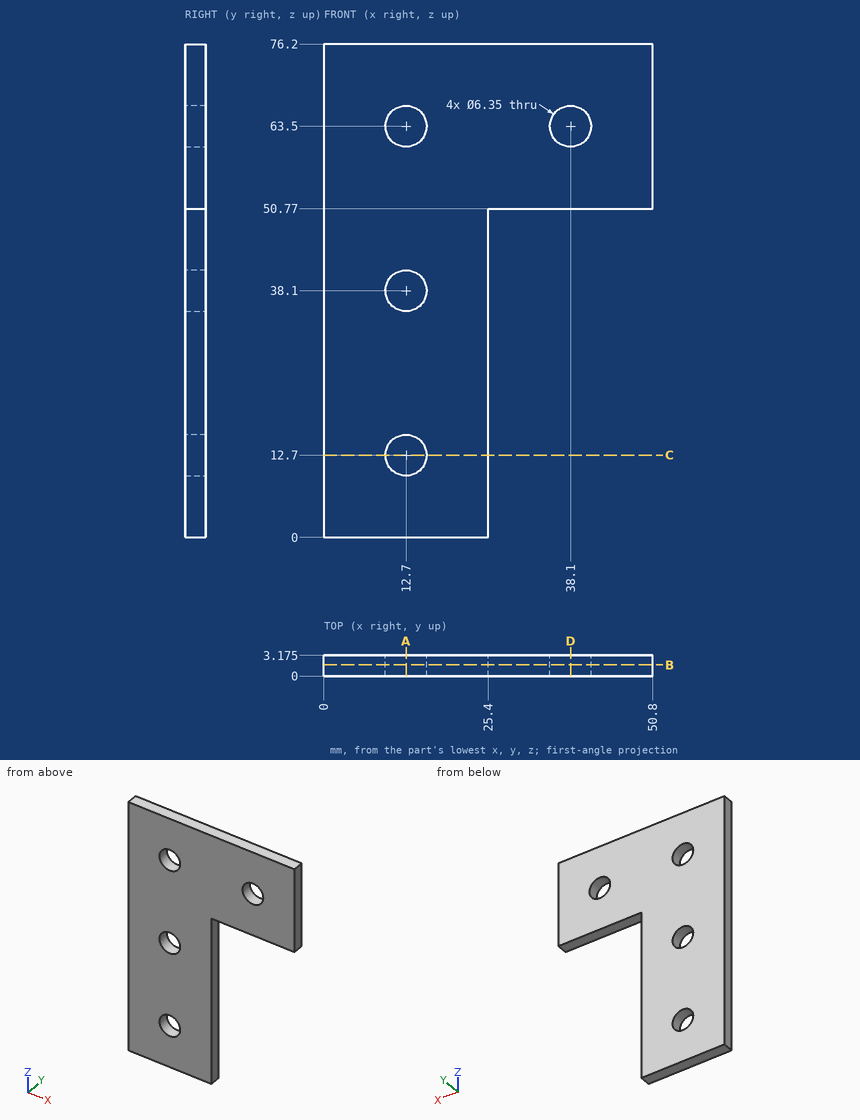
The drawing under review shows one solid part. Ordinate dimensions are in mm from its lowest x, y, z. Round coordinates to 2 decimals unless told otherwise and drop trailing zeros. Loops run counter-clockwise (first coordinate to the right, second up) from the corner with the lowest first, then second, coordinate; pieces in that order, holes last. Notation, with made-up numbers: (43.5, -29) - (92.5, -29) arc R34 cw to (92.5, 7) - close; hole circle Ø3 at (-35.5, 35.5). An arc over 180 degrees is marked (long way). One line per question, with ' | ' between items.
Q1. Take a section at B-B (y = 1.7). State how many separate pieces and enclosed holes the cut face has, and give its area (3 significant figures).
Taken from the geometry:
separate pieces: 1 | enclosed holes: 4 | area: 2,450 mm²
Q2. Take a section at C-C (z = 12.7). Give the boundary of the cut face in (x, y) (1 decimal).
Taken from the geometry:
outline: (0, 0) - (9.5, 0) - (9.5, 3.2) - (0, 3.2) - close; (15.9, 0) - (25.4, 0) - (25.4, 3.2) - (15.9, 3.2) - close
Q3. Take a section at D-D (x = 38.1). Give the boundary of the cut face in (y, z) (1 decimal).
Taken from the geometry:
outline: (0, 50.8) - (3.2, 50.8) - (3.2, 60.3) - (0, 60.3) - close; (0, 66.7) - (3.2, 66.7) - (3.2, 76.2) - (0, 76.2) - close
Q4. For line 1 along X through (y, z) = (0.85, 63.5) (1 decimal); line 2 along X through (y, z) = (1.7, 38.1) (1 decimal); line 3 along Z through (x, y) = (38.1, 2.4) (1 decimal), list the stretches that pass through material, from the lowest coordinate up. Write a range as [from, to].
Taken from the geometry:
line 1: x = [0, 9.5], [15.9, 34.9], [41.3, 50.8] | line 2: x = [0, 9.5], [15.9, 25.4] | line 3: z = [50.8, 60.3], [66.7, 76.2]
Q5. Take a section at A-A (x = 12.7). Give the boundary of the cut face in (y, z) (1 decimal).
Taken from the geometry:
outline: (0, 0) - (3.2, 0) - (3.2, 9.5) - (0, 9.5) - close; (0, 15.9) - (3.2, 15.9) - (3.2, 34.9) - (0, 34.9) - close; (0, 41.3) - (3.2, 41.3) - (3.2, 60.3) - (0, 60.3) - close; (0, 66.7) - (3.2, 66.7) - (3.2, 76.2) - (0, 76.2) - close
Q6. For pin 1 (1.5 mm diameter, centred on x = 33, z = 64.5, fed in from -Y); pin 2 (1.6 mm diameter, centred on y = 1, z = 19.5, fed in from +X), all flat-tipped, find the tip position at first contact; note any pin that passes through.
Taken from the geometry:
pin 1: stops at y = 0 | pin 2: stops at x = 25.4
